```python
from build123d import *

# Parameters (mm, degrees)
CROQUIS1_R              = 1.5
CROQUIS1_W              = 6.2
CROQUIS1_H              = 25
CROQUIS1_H_2            = 15
CROQUIS1_R_2            = 2
CROQUIS1_R_3            = 6.75
CROQUIS1_R_4            = 5.25
CROQUIS1_R_5            = 1.75
SALIENTE_EXTRUIR1_DEPTH = 6


with BuildPart() as part:
    # Croquis1 → Saliente-Extruir1 (new body)
    with BuildSketch(Plane.XY):
        with BuildLine():
            Line((87.635637669, 16), (32.115377174, 16))
            ThreePointArc((32.115377174, 16), (30.701163612, 15.414213562), (30.115377174, 14))
            Line((30.115377174, 14), (30.115377174, 10.910010016))
            Line((30.115377174, 10.910010016), (-30.115377174, 10.910010016))
            Line((-30.115377174, 10.910010016), (-30.115377174, 14))
            ThreePointArc((-30.115377174, 14), (-30.701163612, 15.414213562), (-32.115377174, 16))
            Line((-32.115377174, 16), (-44.664398505, 16))
            Line((-44.664398505, 16), (-87.635637669, 16))
            Line((-87.635637669, 16), (-109, 16))
            ThreePointArc((-109, 16), (-110.414213562, 15.414213562), (-111, 14))
            Line((-111, 14), (-111, 0))
            Line((-111, 0), (-111, -15.999955929))
            ThreePointArc((-111, -15.999955929), (-114.684754838, -37.224148725), (-127.277573278, -54.701697231))
            Line((-127.277573278, -54.701697231), (-135.277573278, -54.701697231))
            Line((-135.277573278, -54.701697231), (-140.277573278, -54.701697231))
            ThreePointArc((-140.277573278, -54.701697231), (-148.762854653, -58.216415857), (-152.277573278, -66.701697231))
            Line((-152.277573278, -66.701697231), (-152.277573278, -303.912438798))
            ThreePointArc((-152.277573278, -303.912438798), (-148.762854653, -312.397720172), (-140.277573278, -315.912438798))
            Line((-140.277573278, -315.912438798), (-135.277573278, -315.912438798))
            Line((-135.277573278, -315.912438798), (-119.364295205, -315.912438798))
            Line((-119.364295205, -315.912438798), (119.364429455, -315.912438798))
            Line((119.364429455, -315.912438798), (130.295105026, -315.912438798))
            Line((130.295105026, -315.912438798), (146.942872896, -315.912438798))
            ThreePointArc((146.942872896, -315.912438798), (155.42815427, -312.397720172), (158.942872896, -303.912438798))
            Line((158.942872896, -303.912438798), (158.942872896, -70.770984471))
            Line((158.942872896, -70.770984471), (158.942872896, -66.701697231))
            ThreePointArc((158.942872896, -66.701697231), (155.42815427, -58.216415857), (146.942872896, -54.701697231))
            Line((146.942872896, -54.701697231), (126.134028278, -54.701697231))
            ThreePointArc((126.134028278, -54.701697231), (114.918041875, -36.777730062), (111, -15.999955929))
            Line((111, -15.999955929), (111, 14))
            ThreePointArc((111, 14), (110.414213562, 15.414213562), (109, 16))
            Line((109, 16), (87.635637669, 16))
        make_face()
        with Locations((-138.277573278, -305.912438798)):
            Circle(CROQUIS1_R, mode=Mode.SUBTRACT)
        with Locations((-95.05, -282.201697231)):
            Rectangle(CROQUIS1_W, CROQUIS1_H, mode=Mode.SUBTRACT)
        with Locations((-95, -239.701697231)):
            Circle(CROQUIS1_R, mode=Mode.SUBTRACT)
        Polygon((-3.049885808, -294.789219369), (-3.049896429, -269.789219369), (3.050103571, -269.789216778), (3.050114192, -294.789216778), align=None, mode=Mode.SUBTRACT)
        with Locations((9.0826e-05, -239.789218073)):
            Circle(CROQUIS1_R, mode=Mode.SUBTRACT)
        with Locations((-95.05, -197.201697231)):
            Rectangle(CROQUIS1_W, CROQUIS1_H, mode=Mode.SUBTRACT)
        with Locations((-95, -154.701697231)):
            Circle(CROQUIS1_R, mode=Mode.SUBTRACT)
        Polygon((-2.949921919, -209.789219327), (-2.94993254, -184.789219327), (3.15006746, -184.789216735), (3.150078081, -209.789216735), align=None, mode=Mode.SUBTRACT)
        with Locations((5.4715e-05, -154.789218073)):
            Circle(CROQUIS1_R, mode=Mode.SUBTRACT)
        Polygon((91.950125201, -294.701658167), (91.95011458, -269.701658167), (98.15011458, -269.701655533), (98.150125201, -294.701655533), align=None, mode=Mode.SUBTRACT)
        with Locations((146.722426722, -305.912438798)):
            Circle(CROQUIS1_R, mode=Mode.SUBTRACT)
        with Locations((95.000101835, -239.701656871)):
            Circle(CROQUIS1_R, mode=Mode.SUBTRACT)
        Polygon((91.95008909, -209.701658167), (91.950078469, -184.701658167), (98.150078469, -184.701655533), (98.15008909, -209.701655533), align=None, mode=Mode.SUBTRACT)
        with Locations((95.000065724, -154.701656871)):
            Circle(CROQUIS1_R, mode=Mode.SUBTRACT)
        with Locations((-95.05, -112.201697231)):
            Rectangle(CROQUIS1_W, CROQUIS1_H, mode=Mode.SUBTRACT)
        with Locations((-95, -69.701697231)):
            Circle(CROQUIS1_R, mode=Mode.SUBTRACT)
        Polygon((-3.04995803, -124.789219369), (-3.049968651, -99.789219369), (3.150031349, -99.789216735), (3.15004197, -124.789216735), align=None, mode=Mode.SUBTRACT)
        with Locations((1.8603e-05, -69.789218073)):
            Circle(CROQUIS1_R, mode=Mode.SUBTRACT)
        with Locations((-138.277573278, -60.912438798)):
            Circle(CROQUIS1_R, mode=Mode.SUBTRACT)
        with Locations((-95.05, -41.5)):
            Rectangle(CROQUIS1_W, CROQUIS1_H_2, mode=Mode.SUBTRACT)
        with Locations((-95, -26)):
            Circle(CROQUIS1_R, mode=Mode.SUBTRACT)
        with Locations((-106.313708499, -11.313708499)):
            Circle(CROQUIS1_R_2, mode=Mode.SUBTRACT)
        with Locations((-83.686291501, -11.313708499)):
            Circle(CROQUIS1_R_2, mode=Mode.SUBTRACT)
        with Locations((-95, 0)):
            Circle(CROQUIS1_R_3, mode=Mode.SUBTRACT)
        with Locations((-106.313708499, 11.313708499)):
            Circle(CROQUIS1_R_2, mode=Mode.SUBTRACT)
        with Locations((-83.686291501, 11.313708499)):
            Circle(CROQUIS1_R_2, mode=Mode.SUBTRACT)
        Polygon((-3.049990229, -48.999960936), (-3.049996601, -33.999960936), (3.150003399, -33.999958302), (3.150009771, -48.999958302), align=None, mode=Mode.SUBTRACT)
        with Locations((0.004600085, -25.999981675)):
            Circle(CROQUIS1_R, mode=Mode.SUBTRACT)
        with Locations((-5.656854249, -5.656854249)):
            Circle(CROQUIS1_R, mode=Mode.SUBTRACT)
        Circle(CROQUIS1_R_4, mode=Mode.SUBTRACT)
        with Locations((-5.656854249, 5.656854249)):
            Circle(CROQUIS1_R, mode=Mode.SUBTRACT)
        Polygon((91.950052978, -124.701658167), (91.950042357, -99.701658167), (98.150042357, -99.701655533), (98.150052978, -124.701655533), align=None, mode=Mode.SUBTRACT)
        with Locations((95.000029612, -69.701656871)):
            Circle(CROQUIS1_R, mode=Mode.SUBTRACT)
        with Locations((5.656854249, -5.656854249)):
            Circle(CROQUIS1_R, mode=Mode.SUBTRACT)
        with Locations((5.656854249, 5.656854249)):
            Circle(CROQUIS1_R, mode=Mode.SUBTRACT)
        with Locations((56.686291501, 11.313708499)):
            Circle(CROQUIS1_R_5, mode=Mode.SUBTRACT)
        Polygon((91.950020817, -48.999960936), (91.950014445, -33.999960936), (98.150014445, -33.999958302), (98.150020817, -48.999958302), align=None, mode=Mode.SUBTRACT)
        with Locations((95.000011046, -25.99995964)):
            Circle(CROQUIS1_R, mode=Mode.SUBTRACT)
        with Locations((146.722426722, -60.912438798)):
            Circle(CROQUIS1_R, mode=Mode.SUBTRACT)
        with Locations((83.686291501, -11.313708499)):
            Circle(CROQUIS1_R_2, mode=Mode.SUBTRACT)
        with Locations((106.313708499, -11.313708499)):
            Circle(CROQUIS1_R_2, mode=Mode.SUBTRACT)
        with Locations((95, 0)):
            Circle(CROQUIS1_R_3, mode=Mode.SUBTRACT)
        with Locations((83.686291501, 11.313708499)):
            Circle(CROQUIS1_R_2, mode=Mode.SUBTRACT)
        with Locations((106.313708499, 11.313708499)):
            Circle(CROQUIS1_R_2, mode=Mode.SUBTRACT)
    extrude(amount=SALIENTE_EXTRUIR1_DEPTH)


solid = part.part
```
The model under review builds one solid part; all positions refer to its coordinate system, in mm. Round coordinates to 2 decimals unless told otherwise and drop trailing zeros. Write each loop counter-clockwise with the first axis right and the second up, starting at its lowest first coordinate (ties: lowest second). Pieces come first, ordered by that corner, then holes. Notation, with made-up numbers: M 8.25,25 L 67.25,25 A10 cw 67.25,39 Z; hole C -10,56.5 d5. An arc over 180 degrees is marked long. Use CSV: the item, a comma, the result in double quotes. Start each with the question number.
(1) The part is to be moulded in two halves that separate along Y. For faces 1 (the face through (155.334, -312.491, 2.958)), 2 (the face through (1, -148, 6)), 3 (the face through (5, 1.6, 3)), say which applies: +Y half, -Y half, draft (parallel to the pull), parting line (faces both ways), or undercut.
(2) For line 1 along X through (y, z) = (-271, 0.75); line 2 along X through (y, z) = (-11, 5.05); line 3 along X through (y, z) = (-37.5, 2.2), list the stretches that pass through material, from the lowest coordinate up.
(3) We need section C-C, the plane y = -116. State the section outline as (x, z) points, then the cut area to 3 significant figures.
(4) We need section B-B, the plane x = -20. State the section outline as (y, z) points, then the cut area to 3 significant figures.
(5) We need section A-A, the plane y = 0. State the section outline as (x, z) points.
(6) Clearance check with flat-ended pins moving along their axes: P1, Ø1.8, axis at x = -133, z = 2, coming from the +Y side; P2, Ø2, axis at x = -26, z = 2.5, coming from the +Y side; P3, Ø3, axis at x = 123, z = 5, coming from the +Y side. State where each tip first meets the part, or that it passes through.
(7) We need section D-D, the plane z = 3.35. State how many separate pieces and enclosed holes the cut face has, then the cut area to 3 significant figures.
Findings:
1,face 1,"-Y half"
1,face 2,"draft"
1,face 3,"undercut"
2,line 1,"-152.28 to -98.15, -91.95 to -3.05, 3.05 to 91.95, 98.15 to 158.94"
2,line 2,"-111 to -108.29, -104.34 to -85.66, -81.71 to 81.71, 85.66 to 104.34, 108.29 to 111"
2,line 3,"-114.8 to -98.15, -91.95 to -3.05, 3.15 to 91.95, 98.15 to 115.21"
3,outline,"M -152.28,0 L -98.15,0 L -98.15,6 L -152.28,6 Z; M -91.95,0 L -3.05,0 L -3.05,6 L -91.95,6 Z; M 3.15,0 L 91.95,0 L 91.95,6 L 3.15,6 Z; M 98.15,0 L 158.94,0 L 158.94,6 L 98.15,6 Z"
3,area,"1,760 mm^2"
4,outline,"M -315.91,0 L 10.91,0 L 10.91,6 L -315.91,6 Z"
4,area,"1,960 mm^2"
5,outline,"M -111,0 L -101.75,0 L -101.75,6 L -111,6 Z; M -88.25,0 L -5.25,0 L -5.25,6 L -88.25,6 Z; M 5.25,0 L 88.25,0 L 88.25,6 L 5.25,6 Z; M 101.75,0 L 111,0 L 111,6 L 101.75,6 Z"
6,P1,"y = -54.7"
6,P2,"y = 10.91"
6,P3,"y = -48.98"
7,separate pieces,"1"
7,enclosed holes,"44"
7,area,"94,600 mm^2"
